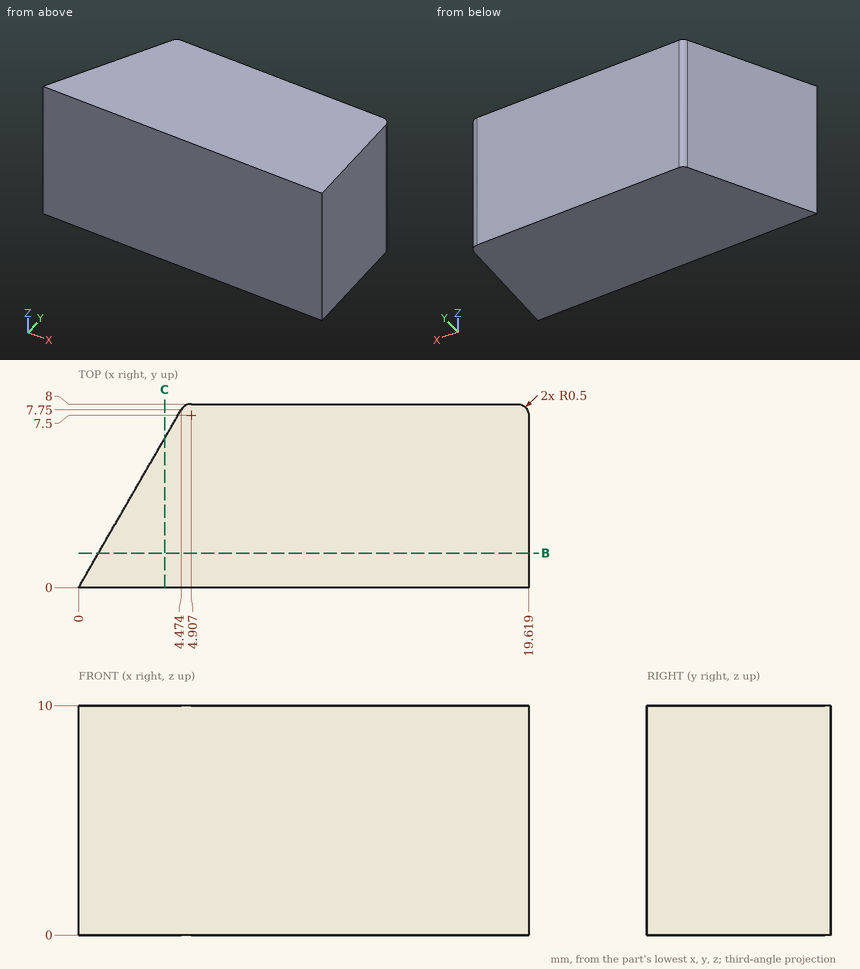
Here's the drawing with two shaded views (mm, measured from the low corner). I have some questions. Round coordinates to 2 decimals unless told otherwise and drop trailing zeros. Order: outer loops, then holes, each group sorted by start corner. A loop starts at its lowest first (then second) coordinate and runs counter-clockwise, first axis right, second up. Notation, with made-up numbers: (79, 80.25) -> (109, 80.25) arc R30 cw to (109, 114.25) -> close; hole circle Ø11 at (57, -10.5). An arc over 180 degrees is marked (long way). Write each question's results on one line, items separated by ' | '. Start each with the question number.
Item 1: Will these pins go through, and if not, where does the flat tip stop? pin 1 (1.5 mm diameter, centred on x = 4, z = 5, fed in from -Y); pin 2 (4 mm diameter, centred on y = 1, z = 6, fed in from -X); pin 3 (1.5 mm diameter, centred on x = 2.5, z = 5.5, fed in from +Y).
Item 2: Please list where these lines run through material, in increasing order: L1, parallel to X at y = 6.75, z = 2.5; L2, parallel to Y at x = 4.5, z = 6.5; L3, parallel to X at y = 4.25, z = 2 (1 decimal).
Item 3: If we section it at C-C, the plane x = 3.75: Write out the boundary of the cut face in (y, z) (1 decimal).
Item 4: If we section it at B-B, the plane y = 1.5: Write out the boundary of the cut face in (x, z).
Results:
1) pin 1: stops at y = 0 | pin 2: stops at x = 0 | pin 3: stops at y = 5.63
2) L1: x = 3.9 to 19.62 | L2: y = 0 to 7.79 | L3: x = 2.5 to 19.6
3) outline: (0, 0) -> (6.5, 0) -> (6.5, 10) -> (0, 10) -> close
4) outline: (0.87, 0) -> (19.62, 0) -> (19.62, 10) -> (0.87, 10) -> close
